Autodesk Inventor part; units mm, degrees
ref_plane "YZ Plane" through (0, 0, 0) normal (1, 0, 0) x (0, 1, 0)
ref_plane "XZ Plane" through (0, 0, 0) normal (0, 1, 0) x (-1, 0, 0)
ref_plane "XY Plane" through (0, 0, 0) normal (0, 0, 1) x (1, 0, 0)
sketch "Sketch2" plane through (0, 0, 0) normal (0, 1, 0) x (-1, 0, 0)
  line L0 (-16, 8) -> (16, 8)
  line L1 (16, 8) -> (16, -8)
  line L2 (16, -8) -> (-16, -8)
  line L3 (-16, -8) -> (-16, 8)
  point P0 (0, 0)
  point P1 (0, 8)
  point P2 (-16, 0)
  dimension "d0" = 32
  dimension "d1" = 16
extrude "Extrusion1" add sketch "Sketch2" along normal blind 9.6
sketch "Sketch10" plane through (0, 0, 0) normal (0, 0, 1) x (1, 0, 0)
  line L0 (-16, 9.6) -> (16, 9.6)
  line L1 (-16, 0) -> (-16, 9.6)
  arc A0 (16, 1.6) -> (-16, 9.6) centre (-16, -58.4) ccw
  line L2 (16, 1.6) -> (16, 9.6)
  line L3 (-16, 0) -> (16, 0)
  line L4 (14.4, 0) -> (14.4, 1.6)
  line L5 (14.4, 1.6) -> (12.4422, 1.6)
  line L6 (-8, 3.2) -> (-8, 7.5163)
  line L7 (-6.4, 7.3024) -> (-6.4, 3.2)
  arc A1 (12.4422, 1.6) -> (-6.4, 7.3024) centre (-16, -58.4) ccw
  arc A2 (-8, 7.5163) -> (-14.4, 7.9807) centre (-16, -58.4) ccw
  line L8 (-14.4, 7.9807) -> (-14.4, 6.4)
  line L9 (1.6, 5.625) -> (1.6, 0)
  line L10 (0, 6.0435) -> (0, 0)
  line L11 (0, 3.2) -> (-6.4, 3.2)
  line L12 (-8, 6.4) -> (-14.4, 6.4)
  line L13 (-14.4, 6.4) -> (-16, 6.4)
  line L14 (16, 0) -> (16, 9.6)
  line L15 (1.6, 0) -> (14.4, 0)
  line L16 (0, 0) -> (-16, 0)
  line L17 (-16, 0) -> (-16, 6.4)
  line L18 (-6.4, 3.2) -> (-8, 3.2)
  dimension "d100" = 1.6
  dimension "d104" = 1.6
  dimension "d105" = 1.6
  dimension "d107" = 1.6
  dimension "d108" = 1.6
  dimension "d113" = 6.4
  dimension "d114" = 3.2
  dimension "d115" = 16
  dimension "d116" = 1.6
extrude "Extrusion7" cut sketch "Sketch10" along normal through all both and the other way through all contours L0 L2 A0 | L13 L12 L6 L18 L11 L10 L3 L1
extrude "Extrusion8" cut sketch "Sketch10" along normal mid plane 12.8 contours L8 A2 L6 L12 | L3 L9 A1 L5 L4 | L11 L7 A1 L10
sketch "Sketch3" plane through (0, 0, 0) normal (0, -1, 0) x (1, 0, 0)
  circle A0 centre (12, 4) radius 2.4 construction
  line L0 (14.4, -6.4) -> (1.6, -6.4)
  line L1 (1.6, -6.4) -> (1.6, 6.4)
  line L2 (1.6, 6.4) -> (14.4, 6.4)
  line L3 (14.4, 6.4) -> (14.4, -6.4)
  circle A1 centre (8, 0) radius 3.2569
  circle A2 centre (8, 0) radius 2.4
  circle A3 centre (12, -4) radius 2.4 construction
  point P0 (8, 6.4)
  point P1 (1.6, 0)
  dimension "d97" = 4.8
extrude "Extrusion2" add sketch "Sketch3" against normal up to next contours A1
sketch "Sketch11" plane through (-8, 3.2, 8) normal (0, -1, 0) x (1, 0, 0)
  line L0 (8, -1.6) -> (8, 0)
  line L1 (8, -14.4) -> (1.6, -14.4)
  line L2 (1.6, -14.4) -> (1.6, -1.6)
  circle A0 centre (4, -12) radius 2.4 construction
  line L3 (8, -11.4) -> (6.4, -11.4)
  line L4 (6.4, -11.4) -> (6.4, -12.6)
  line L5 (6.4, -12.6) -> (8, -12.6)
  line L6 (8, -11.4) -> (8, -12.6)
  line L7 (1.6, -1.6) -> (8, -1.6)
  circle A1 centre (4, -4) radius 2.4 construction
  line L8 (8, -4.6) -> (6.4, -4.6)
  line L9 (6.4, -4.6) -> (6.4, -3.4)
  line L10 (6.4, -3.4) -> (8, -3.4)
  line L11 (8, -3.4) -> (8, -4.6)
  circle A2 centre (4, -8) radius 1.6
  line L12 (6.4, -7.4) -> (8, -7.4)
  line L13 (8, -7.4) -> (8, -8.6)
  line L14 (8, -8.6) -> (6.4, -8.6)
  line L15 (6.4, -8.6) -> (6.4, -7.4)
  point P0 (8, -8)
  point P1 (6.4, -12)
  point P2 (6.4, -4)
  point P3 (6.4, -8)
  dimension "d119" = 1.2
  dimension "d129" = 4.8
extrude "Extrusion9" add sketch "Sketch11" against normal up to next
sketch "Sketch12" plane through (-16, 6.4, 8) normal (0, -1, 0) x (1, 0, 0)
  line L0 (1.6, -1.6) -> (8, -1.6)
  line L1 (8, -14.4) -> (1.6, -14.4)
  line L2 (1.6, -14.4) -> (1.6, -1.6)
  line L3 (8, -3.4) -> (6.4, -3.4)
  line L4 (6.4, -3.4) -> (6.4, -4.6)
  line L5 (6.4, -4.6) -> (8, -4.6)
  line L6 (8, -4.6) -> (8, -3.4)
  circle A0 centre (4, -4) radius 2.4 construction
  circle A1 centre (4, -12) radius 2.4 construction
  line L7 (8, -11.4) -> (6.4, -11.4)
  line L8 (6.4, -11.4) -> (6.4, -12.6)
  line L9 (6.4, -12.6) -> (8, -12.6)
  line L10 (8, -12.6) -> (8, -11.4)
  line L11 (8, -7.4) -> (6.4, -7.4)
  line L12 (6.4, -7.4) -> (6.4, -8.6)
  line L13 (6.4, -8.6) -> (8, -8.6)
  line L14 (8, -8.6) -> (8, -7.4)
  circle A2 centre (4, -8) radius 1.6
  point P0 (16, -8)
  point P1 (6.4, -4)
  point P2 (6.4, -12)
  point P3 (6.4, -8)
  dimension "d122" = 1.2
  dimension "d130" = 4.8
extrude "Extrusion10" add sketch "Sketch12" against normal up to next
fillet "Fillet1" radius 0.1 12 edges at (-16, 8, 8) (-16, 9.6, 0) (16, 0.8, 8) (16, 0.8, -8) (-16, 8, -8) (0.4924, 7.5697, 8) (0.4924, 7.5697, -8) (16, 1.6, 0) (-8, 4.8, 8) (0, 1.6, 8) (0, 1.6, -8) (-8, 4.8, -8)
equation "\"d4\" = lh"
equation "\"d100\" = wall"
equation "\"d104\" = wall"
equation "\"d105\" = 0.333333 * lh - topthk"
equation "\"d107\" = topthk"
equation "\"d108\" = d104"
equation "\"d113\" = 0.666667 * lh"
equation "\"d114\" = 0.333333 * lh"
equation "\"d115\" = 2 * lu"
equation "\"d116\" = wall"
equation "\"d109\" = 2 * lu - 2 * wall"
equation "\"d97\" = kd"
equation "\"d129\" = kd"
properties part number "93606-Black" material "ABS Plastic"
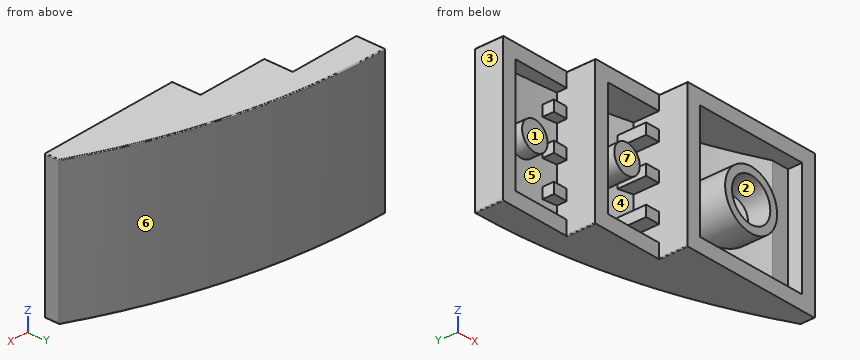
Here's how the part is built. I have some questions about the finished solid (model axes, mm). Face numbers are marked on the shaded views. A direction names the side the tool comes from. Round coordinates to 2 decimals unless told otherwise and drop trailing zeros.
Q1. Please list where these lines run through material, in increasing order: probe 1 along X at (y, z) = (1.35, 0); probe 2 along Z at (x, y) = (8, 1.9); probe 3 along X at (y, z) = (2.45, 0).
Q2. Which directions (+Z, -Z, +X, -X, +Y, -Y) give clear straight access to the entire face, cutting with the end or side of a thin tool? Please do the marked faces 1, 2 and 3.
Q3. Will these pins go through, and if not, where does the flat tip stop? P1, Ø1.3, axis at y = 5.5, z = -1.5, coming from the -X side; P2, Ø1, axis at x = -12.5, z = 1, coming from the -Y side; P3, Ø4, axis at y = 4, z = 1.5, coming from the +X side; P4, Ø2, axis at y = 6, z = 1, coming from the -X side.
Q4. If we mould it in two halves opening along X, with no side actions, what happens to the marked faces 4, 5, 6 and 7? For each: +X half, -X half, draft (parallel to the pull), parting line (faces both ways), or undercut.
Answer below:
1. probe 1: x = 0 to 1.6, 4.74 to 5.6, 10.4 to 11.26, 14.4 to 16
1. probe 2: z = -8 to -6.4, -3.26 to -2.4, 2.4 to 3.26, 6.4 to 8
1. probe 3: x = 0 to 1.6, 4.74 to 5.6, 10.4 to 14.35
2. face 1: +Z, -Z, -X, -Y
2. face 2: -Y
2. face 3: +Z, -Z, -X, +Y, -Y
3. P1: stops at x = -8
3. P2: stops at y = 6.4
3. P3: stops at x = 15.24
3. P4: stops at x = -16
4. face 4: undercut
4. face 5: undercut
4. face 6: +X half
4. face 7: draft
